Work out the finished part from the listing and answer in its coordinate system (mm). A direction names the side the tool comes from. Coordinates: 2 decimals unless noted, no trailing zeros. Order: outer loops, then holes, each group sorted by start corner. A loop starts at its lowest first (then second) coordinate and runs counter-clockwise, first axis right, second up. Notation, with made-up numbers: (-20, -31.75) -> (26, -31.75) arc R27 ccw to (26, 6.25) -> close; hole circle Ø11 at (31, 14.5). An arc over 180 degrees is marked (long way). Answer as CSV lines item,"result". Start each with the question number.
Item 1: For a pull along Z with two mould halves and no side action, classify faces 3 (the face through (-57.138, -76.911, 1.186)), 4 (the face through (-13.77, -62.61, -61.99)), 5 (the face through (0, -127, 0)) as pulls with the +Z half, pulls with the -Z half, needs draft (parallel to the pull), parting line crosses it, or undercut.
Item 2: Each of these flat-tipped pins is pushed along its axis until it touches: pin 1 Ø5 at (y, z) = (-16.5, -27) entering from +X; pin 2 Ø5 at (y, z) = (-82.5, -23) entering from +X; pin 3 Ø2 at (x, z) = (-20, -30) entering from -Y. Where does it stop, or does it pass through?
Item 3: Section D-D (z = 53.5) is taken. Write down the section's boundary in (x, y).
Item 4: Section A-A (y = -66.5) is taken. Write down the section's boundary in (x, z), then the cut area to 3 significant figures.
Item 5: Straight lines are drawn through the part: L1, parallel to X at y = -110, z = 2 (1 decimal); L2, parallel to X at y = -105, z = -12; L3, parallel to Y at x = -45.5, z = -31. For each, find the intervals that lie inside material, in ascending order.
Item 6: Section C-C (x = 7) is taken. Write down the section's boundary in (y, z).
Item 7: Which of the six approach directions +Z, -Z, +X, -X, +Y, -Y give full straight-line access (tool end or side, diameter ignored) to faces 1 (the face through (-1, 0, 1)), 2 (the face through (5.063, -75, -1))?
Item 8: Section B-B (z = 0) is taken. Write down the section's boundary in (x, y).
```python
from build123d import *

# Parameters (mm, degrees)
F0_R     = 63.5
F1_DEPTH = 127
F4_D     = 114.3
F5_DEPTH = 25.4
F6_W     = 10.1255085319
F6_H     = 120.7859069109
F7_DEPTH = 101.6


# Not quite as in the source:
# - a feature names something its author has since deleted; it is built from what else it names


with BuildPart() as f1:
    # F0 (on Front) → F1 (new body)
    with BuildSketch(Plane.XZ):
        Circle(F0_R)
    extrude(amount=F1_DEPTH)

    # F4 (through all)
    with Locations(Plane(origin=(0, 0, 0), x_dir=(-1, 0, 0), z_dir=(0, 1, 0))):
        with Locations((0, 0)):
            Hole(F4_D / 2)

    # F0 (on Front) → F5 (join)
    with BuildSketch(Plane.XZ):
        Circle(F0_R)
    extrude(amount=F5_DEPTH)

    # F6 (on face) → F7 (join)
    with BuildSketch(Plane.XZ.offset(25.4)):
        Rectangle(F6_W, F6_H)
    extrude(amount=F7_DEPTH)


solid = f1.part
```
Checked values:
1,face 3,"undercut"
1,face 4,"parting line crosses it"
1,face 5,"needs draft"
2,pin 1,"stops at x = 58.58"
2,pin 2,"stops at x = 60.1"
2,pin 3,"stops at y = -25.4"
3,outline,"(-34.21, -127) -> (-20.1, -127) -> (-20.1, -25.4) -> (-5.06, -25.4) -> (-5.06, -127) -> (5.06, -127) -> (5.06, -25.4) -> (20.1, -25.4) -> (20.1, -127) -> (34.21, -127) -> (34.21, 0) -> (-34.21, 0) -> close"
4,outline,"circle Ø127 at (0, 0); hole (-5.06, -56.93) -> (-5.06, 56.93) arc R57.15 ccw to start; hole (5.06, -56.93) arc R57.15 ccw to (5.06, 56.93) -> close"
4,area,"3,560 mm^2"
5,L1,"x = -63.5 to -57.1, -5.1 to 5.1, 57.1 to 63.5"
5,L2,"x = -62.36 to -55.88, -5.06 to 5.06, 55.88 to 62.36"
5,L3,"y = -25.4 to 0"
6,outline,"(-127, -63.11) -> (0, -63.11) -> (0, 63.11) -> (-127, 63.11) -> (-127, 56.72) -> (-25.4, 56.72) -> (-25.4, -56.72) -> (-127, -56.72) -> close"
7,face 1,"+Z, -Z, +X, -X, +Y"
7,face 2,"-Y"
8,outline,"(-63.5, -127) -> (-57.15, -127) -> (-57.15, -25.4) -> (-5.06, -25.4) -> (-5.06, -127) -> (5.06, -127) -> (5.06, -25.4) -> (57.15, -25.4) -> (57.15, -127) -> (63.5, -127) -> (63.5, 0) -> (-63.5, 0) -> close"
